from build123d import *

# Parameters (mm, degrees)
PROFILE_SKETCH_W      = 14.25
PROFILE_SKETCH_H      = 7.4
PROFILE_SKETCH_W_2    = 9.25
PROFILE_SKETCH_H_2    = 2.4
PROFILE_EXTRUDE_DEPTH = 15
CORNER_FILLETS_R      = 2


with BuildPart() as part:
    # Profile Sketch → Profile Extrude (new body)
    with BuildSketch(Plane.XY):
        Rectangle(PROFILE_SKETCH_W, PROFILE_SKETCH_H)
        Rectangle(PROFILE_SKETCH_W_2, PROFILE_SKETCH_H_2, mode=Mode.SUBTRACT)
    extrude(amount=PROFILE_EXTRUDE_DEPTH)

    # Corner Fillets
    corner_fillets_edges = [part.edges().sort_by_distance(p)[0] for p in [
        (-7.125, 0, 15),
        (7.125, 0, 15),
        (-7.125, 0, 0),
        (7.125, 0, 0),
    ]]
    fillet(corner_fillets_edges, radius=CORNER_FILLETS_R)


solid = part.part
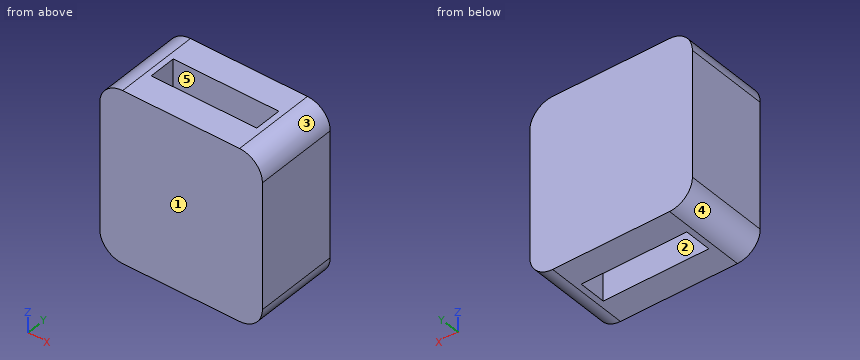
Geometry: final body of the model. Coordinates: model frame, mm. Face numbers are marked on the shaded views. A direction names the side the tool comes from. Coordinates: 2 decimals unless noted, no trailing zeros. Order: outer loops, then holes, each group sorted by start corner. A loop starts at its lowest first (then second) coordinate and runs counter-clockwise, first axis right, second up.
(1) Section query B-B (x = 2.5). Return the cut outline in (y, z).
(2) Access query for the marked faces 4 and 5. Directions: +Z, -Z, +X, -X, +Y, -Y. A direction counts if a zero-diameter tool reaches every point of the face in a straight line with its end or side. Return the directions, or none.
(3) Section query C-C (z = 12). Return the cut outline in (x, y) (3 decimals).
(4) First-contact query: pin 1 (1 mm diameter, centred on x = 5.5, y = -0.5, fed in from +Z). Flat tip, straight axial feed; report the tip coordinate or a pass-through.
(5) Section query A-A (y = 0). Return the cut outline in (x, z) (3 decimals), plus the area to 3 significant figures.
(6) Material intervals for probe 1 along X at (y, z) = (1, 5) (3 decimals); probe 2 along Y at (x, z) = (1.5, 7.75); probe 3 along Z at (x, y) = (-6.25, 2.5), sorted ascending.
(7) Draft query along X for the marked faces 1, 2 and 3. Return one class per face: pulls with the +X half, pulls with the -X half, needs draft (parallel to the pull), parting line crosses it, or undercut.
(8) Section query D-D (y = -1.75). Return the cut outline in (x, z) (3 decimals), plus the area to 3 significant figures.
Solution:
1. outline: (-3.7, 0) - (-1.2, 0) - (-1.2, 15) - (-3.7, 15) - close; (1.2, 0) - (3.7, 0) - (3.7, 15) - (1.2, 15) - close
2. face 4: -Z, -X, +Y, -Y
2. face 5: +Z, -Z
3. outline: (-7.125, -3.7) - (7.125, -3.7) - (7.125, 3.7) - (-7.125, 3.7) - close; hole (-4.625, -1.2) - (4.625, -1.2) - (4.625, 1.2) - (-4.625, 1.2) - close
4. pin 1: stops at z = 15
5. outline: (-7.125, 2) arc R2 ccw to (-5.125, 0) - (-4.625, 0) - (-4.625, 15) - (-5.125, 15) arc R2 ccw to (-7.125, 13) - close; (4.625, 0) - (5.125, 0) arc R2 ccw to (7.125, 2) - (7.125, 13) arc R2 ccw to (5.125, 15) - (4.625, 15) - close
5. area: 71.6 mm2
6. probe 1: x = -7.125 to -4.625, 4.625 to 7.125
6. probe 2: y = -3.7 to -1.2, 1.2 to 3.7
6. probe 3: z = 0.35 to 14.65
7. face 1: needs draft
7. face 2: undercut
7. face 3: pulls with the +X half
8. outline: (-7.125, 2) arc R2 ccw to (-5.125, 0) - (5.125, 0) arc R2 ccw to (7.125, 2) - (7.125, 13) arc R2 ccw to (5.125, 15) - (-5.125, 15) arc R2 ccw to (-7.125, 13) - close
8. area: 210 mm2
